Input: part model. Units: mm. Frame: model coordinates. Round coordinates to 2 decimals unless told otherwise and drop trailing zeros. Loops run counter-clockwise (first coordinate to the right, second up) from the corner with the lowest first, then second, coordinate; pieces in that order, holes last.
1) Section A-A, the plane x = 8. Return loops of the section in (y, z).
2) Ray query, line 1 along Y through (x, z) = (4.75, -0.05); line 2 along Z through (x, y) = (6, 0.5); line 3 along Z through (x, y) = (8.75, 0.55). Return the intervals inside material, ascending.
3) Section D-D, the plane x = 4.5. Return loops of the section in (y, z), and give its area (3 significant figures).
4) Section B-B, the plane y = 0. Return loops of the section in (x, z) (3 decimals), and give its area (3 significant figures).
5) Section C-C, the plane z = 0.4. Return loops of the section in (x, y) (3 decimals), and give its area (3 significant figures).
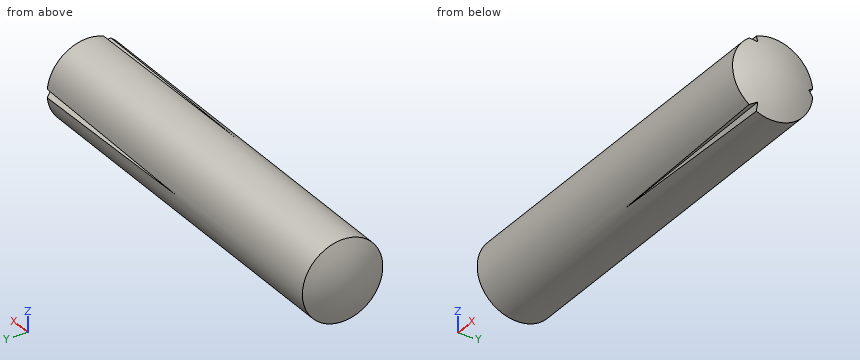
Autodesk Inventor part; units mm, degrees
ref_plane "Work Plane1" through (10, 0, 0) normal (1, 0, 0) x (0, 1, 0)
ref_plane "Work Plane2" through (10, 0, -10) normal (0.9995, -0.032, 0) x (0.032, 0.9995, 0)
ref_plane "YZ Plane" through (0, 0, 0) normal (1, 0, 0) x (0, 1, 0)
sketch "Skizze1" plane through (0, 0, 0) normal (0, 0, 1) x (1, 0, 0)
  line L0 (0, 0) -> (10, 0)
  line L1 (0.25, 1) -> (9.75, 1)
  arc A0 (0.25, 1) -> (0, 0) centre (2.125, 0) ccw
  arc A1 (10, 0) -> (9.75, 1) centre (7.875, 0) ccw
  line L2 (10, 0) -> (10, 0.84) construction
  line L3 (10, 0.84) -> (5, 1) construction
  line L4 (-12.8617, 0) -> (72.8617, 0)
  line L5 (0, 12.1847) -> (0, -2.0308)
  point P0 (5, 0)
  dimension "d0" = 2
  dimension "d1" = 10
  dimension "d2" = 1.68
  dimension "d12" = 5
  dimension "d17" = 0.25
  dimension "d18" = 0.25
revolve "Körper" add sketch "Skizze1" angle 360 about axis through (0, 0, 0) along (1, 0, 0)
ref_plane "Work Plane1" through (10, 0, 0) normal (1, 0, 0) x (0, 1, 0)
sketch "Skizze2" plane through (10, 0, 0) normal (1, 0, 0) x (0, 1, 0)
  line L0 (0, -14) -> (0, 14)
ref_plane "Work Plane2" through (10, 0, -10) normal (0.9995, -0.032, 0) x (0.032, 0.9995, 0)
sketch "Skizze3" plane through (10, 0, -10) normal (0.9995, -0.032, 0) x (0.032, 0.9995, 0)
  ellipse E0 centre (-0.008, 10) end of major axis (-0.008, 11) minor radius 0.9995
  line L0 (-0.1599, 10) -> (0.8396, 10)
  line L1 (0.8396, 10) -> (0.9862, 10.1027)
  line L2 (0.8396, 10) -> (0.9862, 9.8973)
  arc A0 (0.9862, 9.8973) -> (0.9862, 10.1027) centre (-0.008, 10) ccw
  dimension "d7" = 70
extrude "Nut" cut sketch "Skizze3" against normal up to next contours L2 L1 E0 picked at (0.9387, 9.9486)
pattern_circular "Nuten" count 3 over 360 about axis through (5, 0, 0) along (1, 0, 0) of "Nut"
equation "\"d0\" = NND"
equation "\"d1\" = NLG"
equation "\"d2\" = 0.84 * NND"
equation "\"d18\" = KAH"
equation "\"d8\" = 0.5 * NLG"
equation "\"NND\" = 2"
equation "\"NLG\" = 10"
equation "\"KAH\" = 0.25"
equation "\"d6\" = -d5"
equation "\"FAC\" = 0.5"
equation "\"NND1\" = 2.15"
equation "\"NLG1\" = 9.5"
properties part number "ISO 8745 - 2 x 10" material "Edelstahl, austenitisch"
Final values:
1. outline: (-0.56, -0.83) - (-0.45, -0.78) - (-0.44, -0.9) arc R1 ccw to (1, -0.07) - (0.9, 0) - (1, 0.07) arc R1 ccw to (-0.44, 0.9) - (-0.45, 0.78) - (-0.56, 0.83) arc R1 ccw to start
2. line 1: y = -1 to 1
2. line 2: z = -0.87 to 0.87
2. line 3: z = -0.84 to 0.84
3. outline: circle Ø2 at (0, 0)
3. area: 3.14 mm2
4. outline: (0.25, -1) - (9.75, -1) arc R2.125 ccw to (9.75, 1) - (0.25, 1) arc R2.125 ccw to start
4. area: 19.7 mm2
5. outline: (0.25, -0.917) - (9.75, -0.917) arc R2.087 ccw to (9.75, 0.917) - (0.25, 0.917) arc R2.087 ccw to start
5. area: 17.9 mm2
